from build123d import *

# Parameters (mm, degrees)
F0_R           = 37.2422807911
F1_DEPTH       = 25.4
F2_R           = 18.2238332667
F3_DEPTH       = 25.4
F5_D           = 7.9375
F5_CSINK_D     = 19.8374
F5_CSINK_ANGLE = 82


with BuildPart() as f1:
    # F0 (on Top) → F1 (new body)
    with BuildSketch(Plane.XY):
        Circle(F0_R)
    extrude(amount=F1_DEPTH)

    # F2 (on face) → F3 (join)
    with BuildSketch(Plane.XY.offset(25.4)):
        Circle(F2_R)
    extrude(amount=F3_DEPTH)

    # F5 (through all)
    with Locations(Plane.XY.offset(50.8)):
        with Locations((0, 0)):
            CounterSinkHole(F5_D / 2, F5_CSINK_D / 2, counter_sink_angle=F5_CSINK_ANGLE)


solid = f1.part
Input: part model. Units: mm. Frame: model coordinates. A direction names the side the tool comes from. Give positions to 0.01 mm unless a question says otherwise; leave off trailing zeros. Write each loop counter-clockwise with the first axis right and the second up, starting at its lowest first coordinate (ties: lowest second). Pieces come first, ordered by that corner, then holes. Notation, with made-up numbers: M -9.5,-15.75 L 49.5,-15.75 A17 ccw 49.5,15.25 Z; hole C 8.5,87.25 d10. An arc over 180 degrees is marked long. Use one line per item in the form item = value.
1. Mould query, pull axis Y, two halves, no side actions, for faces 1 (the face through (-14.46, -11.09, 37.92)), 2 (the face through (8, 1, 0)), 3 (the face through (3.38, -2.59, 44.29)). Classes: released by +Y, released by -Y, zero draft, split by the parting line, or undercut.
Outcome:
face_1 = split by the parting line
face_2 = zero draft
face_3 = undercut
2. Reachability of faces 4 (the face through (8, 17, 25.4)), 5 (the face through (35.52, 11.19, 12.52)) from +Z, -Z, +X, -X, +Y, -Y: full face, straight path, thin tool, end or side. Return the list, or none.
Outcome:
face_4 = +Z
face_5 = +Z, -Z
3. First-contact query: P1, Ø2, axis at x = 15, z = 12.5, coming from the -Y side; P2, Ø1, axis at y = -1.5, z = 42.5, coming from the +X side; P3, Ø2, axis at y = -7, z = 23.5, coming from the -X side. Flat tips, straight axial feed; report the tip coordinate or a pass-through.
Outcome:
P1 = -34.51
P2 = 18.2
P3 = -36.76
4. Ray query, L1, parallel to Y at x = 0, z = 20.5; L2, parallel to Z at x = -16.5, y = -24; L3, parallel to X at y = 1.5, z = 32.5. Return the intervals inside material, ascending.
Outcome:
L1 = -37.24 to -3.97, 3.97 to 37.24
L2 = 0 to 25.4
L3 = -18.16 to -3.67, 3.67 to 18.16
5. Cut plane D-D on x = 11. Return loops of the section in (y, z), and give its area (3 significant figures).
Outcome:
outline = M -35.58,0 L 35.58,0 L 35.58,25.4 L 14.53,25.4 L 14.53,50.8 L -14.53,50.8 L -14.53,25.4 L -35.58,25.4 Z
area = 2,550 mm²
6. Cut plane C-C on z = 13. Return loops of the section in (x, y), and give its area (3 significant figures).
Outcome:
outline = C 0,0 d74.48; hole C 0,0 d7.94
area = 4,310 mm²
7. Cut plane A-A on x = 0. Return loops of the section in (y, z).
Outcome:
outline = M -37.24,0 L -3.97,0 L -3.97,43.96 L -9.92,50.8 L -18.22,50.8 L -18.22,25.4 L -37.24,25.4 Z; M 3.97,0 L 37.24,0 L 37.24,25.4 L 18.22,25.4 L 18.22,50.8 L 9.92,50.8 L 3.97,43.96 Z
